from build123d import *

# Parameters (mm, degrees)
SKETCH_1_W          = 135
SKETCH_1_H          = 100
SKETCH_1_R          = 1.6
EXTRUDE_1_DEPTH     = 2
SKETCH_2_W          = 10
SKETCH_2_H          = 9
EXTRUDE_2_DEPTH     = 5
SKETCH_3_W          = 115
SKETCH_3_H          = 7
EXTRUDE_3_DEPTH     = 9
SKETCH_4_W          = 7
SKETCH_4_H          = 77
EXTRUDE_4_DEPTH     = 9
SKETCH_5_W          = 49
SKETCH_5_H          = 8
EXTRUDE_5_DEPTH     = 9
SKETCH_6_W          = 25.5
SKETCH_6_H          = 25.5
EXTRUDE_6_DEPTH     = 11
SKETCH_6_5_R        = 4.25
EXTRUDE_10_DEPTH    = 11
SKETCH_6_6_W        = 14
SKETCH_6_6_H        = 14
EXTRUDE_11_DEPTH    = 18.5
SKETCH_8_W          = 21
SKETCH_8_H          = 5
EXTRUDE_12_DEPTH    = 6
SKETCH_9_W          = 7.4
SKETCH_9_H          = 3.2
CUT_EXTRUDE_1_DEPTH = 6


with BuildPart() as part:
    # Sketch 1 → Extrude 1 (new body)
    with BuildSketch(Plane.XY):
        with Locations((67.5, -50)):
            Rectangle(SKETCH_1_W, SKETCH_1_H)
        with Locations((6.5, -6.5)):
            Circle(SKETCH_1_R, mode=Mode.SUBTRACT)
        with Locations((128.5, -6.5)):
            Circle(SKETCH_1_R, mode=Mode.SUBTRACT)
        with Locations((6.5, -93.5)):
            Circle(SKETCH_1_R, mode=Mode.SUBTRACT)
        with Locations((128.5, -93.5)):
            Circle(SKETCH_1_R, mode=Mode.SUBTRACT)
    extrude(amount=EXTRUDE_1_DEPTH)

    # Sketch 2 → Extrude 2 (add)
    with BuildSketch(Plane.XY.offset(2)):
        with Locations((14.5, -95.5)):
            Rectangle(SKETCH_2_W, SKETCH_2_H)
    extrude(amount=EXTRUDE_2_DEPTH)

    # Sketch 3 → Extrude 3 (add)
    with BuildSketch(Plane.XY.offset(2)):
        with Locations((67.5, -3.5)):
            Rectangle(SKETCH_3_W, SKETCH_3_H)
    extrude(amount=EXTRUDE_3_DEPTH)

    # Sketch 4 → Extrude 4 (add)
    with BuildSketch(Plane.XY.offset(2)):
        with Locations((131.5, -48.5)):
            Rectangle(SKETCH_4_W, SKETCH_4_H)
    extrude(amount=EXTRUDE_4_DEPTH)

    # Sketch 5 → Extrude 5 (add)
    with BuildSketch(Plane.XY.offset(2)):
        with Locations((75, -96)):
            Rectangle(SKETCH_5_W, SKETCH_5_H)
    extrude(amount=EXTRUDE_5_DEPTH)

    # Sketch 6 → Extrude 6 (add)
    with BuildSketch(Plane.XY.offset(2)):
        with Locations((13.25, -34.25)):
            Rectangle(SKETCH_6_W, SKETCH_6_H)
    extrude(amount=EXTRUDE_6_DEPTH)

    # Sketch 6_5 → Extrude 10 (add)
    with BuildSketch(Plane.XY.offset(2)):
        with Locations((30.5, -27.25)):
            Circle(SKETCH_6_5_R)
        with Locations((30.5, -41.25)):
            Circle(SKETCH_6_5_R)
        with Locations(Location((4.25, -60.5, 0), (0, 0, 180))):
            Circle(SKETCH_6_5_R)
        with Locations(Location((4.25, -51.5, 0), (0, 0, 180))):
            Circle(SKETCH_6_5_R)
    extrude(amount=EXTRUDE_10_DEPTH)

    # Sketch 6_6 → Extrude 11 (add)
    with BuildSketch(Plane.XY.offset(2)):
        with Locations((7, -72.5)):
            Rectangle(SKETCH_6_6_W, SKETCH_6_6_H)
    extrude(amount=EXTRUDE_11_DEPTH)

    # Sketch 8 → Extrude 12 (add)
    with BuildSketch(Plane.XY.offset(2)):
        with Locations((61.5, -64)):
            Rectangle(SKETCH_8_W, SKETCH_8_H)
        with Locations((91.5, -64)):
            Rectangle(SKETCH_8_W, SKETCH_8_H)
    extrude(amount=EXTRUDE_12_DEPTH)

    # Sketch 9 → Cut-Extrude 1 (cut)
    with BuildSketch(Plane.XZ.offset(100)):
        with Locations((14.5, 4.1)):
            Rectangle(SKETCH_9_W, SKETCH_9_H)
    extrude(amount=-CUT_EXTRUDE_1_DEPTH, mode=Mode.SUBTRACT)


solid = part.part
The model under review builds one solid part; all positions refer to its coordinate system, in mm. A direction names the side the tool comes from. Round coordinates to 2 decimals unless told otherwise and drop trailing zeros. Write each loop counter-clockwise with the first axis right and the second up, starting at its lowest first coordinate (ties: lowest second). Pieces come first, ordered by that corner, then holes. Notation, with made-up numbers: (-21.5, 57) - (9.5, 57) arc R6 ccw to (9.5, 68) - close; hole circle Ø9 at (39.25, 74.5). An arc over 180 degrees is marked (long way). One line per item, written item: value. Start each with the question number.
1. Consider section B-B on y = -16. Write out the cut boundary in (x, z), and give its area (3 significant figures).
2. Clearance check with flat-ended pins moving along their axes: P1, Ø6, axis at x = 18.5, y = -84, coming from the +Z side; P2, Ø4, axis at y = -64, z = 4.5, coming from the -X side; P3, Ø2.5, axis at x = 74, y = -97.5, coming from the +Z side; P4, Ø4, axis at y = -95.5, z = 5.5, coming from the +X side. State where each tip first meets the part, or that it passes through.
3. To check wall thickness, follow L1, parallel to X at y = -93.5, z = 0.9; L2, parallel to Y at x = 82, z = 4.25; L3, parallel to Y at x = 6.5, z = 0.55. State the ranges of each line that lie inside material, in increasing order. Write a range as from..to.
4. Consider section A-A on x = 115. Write out the cut boundary in (y, z).
5. Consider section C-C on z = 4. State how many separate pieces and enclosed holes the cut face has, and give its area (3 significant figures).
6. Consider section D-D on z = 18.5. Write out the cut boundary in (x, y).
7. The part is to be moulded in two halves that separate along X. For faces 1 (the face through (67, -3, 11)), 2 (the face through (129.98, -7.11, 0.99)), say which applies: released by +X, released by -X, zero draft, split by the parting line, or undercut.
8. Machinability: for faces 3 (the face through (91, -64, 8)), 4 (the face through (14, -97, 2.5)), 5 (the face through (4, -61, 13)), which of the approach directions +Z, -Z, +X, -X, +Y, -Y give a long, thin tool a straight path to every point of the face, cutting with its end or side? Answer none if there is none.
Checks:
1. outline: (0, 0) - (135, 0) - (135, 11) - (128, 11) - (128, 2) - (0, 2) - close
1. area: 333 mm^2
2. P1: stops at z = 2
2. P2: stops at x = 0
2. P3: stops at z = 11
2. P4: stops at x = 99.5
3. L1: x = 0..4.9, 8.1..126.9, 130.1..135
3. L2: y = -100..-92, -66.5..-61.5, -7..0
3. L3: y = -100..-95.1, -91.9..-8.1, -4.9..0
4. outline: (-100, 0) - (0, 0) - (0, 11) - (-7, 11) - (-7, 2) - (-100, 2) - close
5. separate pieces: 12
5. enclosed holes: 0
5. area: 3,060 mm^2
6. outline: (0, -79.5) - (14, -79.5) - (14, -65.5) - (0, -65.5) - close
7. face 1: zero draft
7. face 2: undercut
8. face 3: +Z
8. face 4: -Y
8. face 5: +Z, +X, -X, +Y
